```python
from build123d import *

# Parameters (mm, degrees)
M3_SFHCS_IN_HAV_A1_D           = 3.4
M3_SFHCS_IN_HAV_A1_CSINK_D     = 6.72
M3_SFHCS_IN_HAV_A1_CSINK_ANGLE = 90
DAIRESEL_KAPLAMA1_COUNT        = 10


with BuildPart() as part:
    # Çizim1 → Döndür2 (revolve)
    with BuildSketch(Plane.XY, mode=Mode.PRIVATE) as d_nd_r2_sk:
        with BuildLine():
            Line((26.6, -13.648391358), (26.6, -3.648391358))
            Line((26.6, -3.648391358), (25.1, -3.648391358))
            Line((25.1, -3.648391358), (25.1, 4.751608642))
            ThreePointArc((25.1, 4.751608642), (30.108474042, 16.843134601), (42.2, 21.851608642))
            Line((42.2, 21.851608642), (55.5, 21.851608642))
            ThreePointArc((55.5, 21.851608642), (60.449747468, 23.901861174), (62.5, 28.851608642))
            Line((62.5, 28.851608642), (62.5, 53.351608642))
            Line((62.5, 53.351608642), (64, 53.351608642))
            Line((64, 53.351608642), (64, 61.351608642))
            Line((64, 61.351608642), (66, 61.351608642))
            Line((66, 61.351608642), (66, 51.351608642))
            Line((66, 51.351608642), (64.5, 51.351608642))
            Line((64.5, 51.351608642), (64.5, 18.851608642))
            Line((64.5, 18.851608642), (39.98, 18.851608642))
            ThreePointArc((39.98, 18.851608642), (31.57957144, 15.372037203), (28.1, 6.971608642))
            Line((28.1, 6.971608642), (28.1, -13.648391358))
            Line((28.1, -13.648391358), (26.6, -13.648391358))
        make_face()
    revolve(d_nd_r2_sk.sketch.rotate(Axis((0, 0, 0), (0, 1, 0)), 90), axis=Axis((0, 0, 0), (0, 1, 0)))

    # M3 SFHCS İçin Havşa1 (through all)
    with Locations(Plane(origin=(8.5, 18.851608642, 50.5), x_dir=(0, 0, -1), z_dir=(0, -1, 0))):
        with Locations((0, 0)):
            m3_sfhcs_in_hav_a1 = CounterSinkHole(M3_SFHCS_IN_HAV_A1_D / 2, M3_SFHCS_IN_HAV_A1_CSINK_D / 2, counter_sink_angle=M3_SFHCS_IN_HAV_A1_CSINK_ANGLE)

    # Dairesel Kaplama1: M3 SFHCS İçin Havşa1 ×10 about axis
    dairesel_kaplama1_axis = Axis((0, 0, 0), (0, 1, 0))
    for i in range(1, DAIRESEL_KAPLAMA1_COUNT):
        add(m3_sfhcs_in_hav_a1.rotate(dairesel_kaplama1_axis, i * 360 / DAIRESEL_KAPLAMA1_COUNT), mode=Mode.SUBTRACT)


solid = part.part
```
Read the model definition and answer for the solid it produces. Units are mm, in the model's axes. A direction names the side the tool comes from. Give positions to 0.01 mm unless a question says otherwise; leave off trailing zeros. Order: outer loops, then holes, each group sorted by start corner. A loop starts at its lowest first (then second) coordinate and runs counter-clockwise, first axis right, second up.
(1) Straight lines are drawn through the part: L1, parallel to X at y = 40.5, z = 0; L2, parallel to X at y = 0.5, z = 0; L3, parallel to Y at x = 30, z = 40. For each, find the intervals that lie inside material, in ascending order.
(2) Given pin 1 (12 mm diameter, centred on x = 46, z = -50, fed in from +Y); pin 2 (3 mm diameter, centred on x = -45.4, z = 23.69, fed in from -Y); pin 3 (4 mm diameter, centred on x = 45.4, z = -23.69, fed in from +Y); pin 4 (1.5 mm diameter, centred on x = -39, z = 16, fed in from -Y), each flat-ended and moving along its own axis, determine where each tip first touches the part or whether it passes through.
(3) Find section D-D (y = 34.5). Give the vertices of the cut face in (x, z), plus the area to 3 significant figures.
(4) For faces 4 (the cylindrical face through (-2.75, 41.27, 62.44)), 5 (the cylindrical face through (9.613, 0.61, -23.186)), 6 (the flat face through (14.4, 51.352, -63.2)), determine the directions among +Z, -Z, +X, -X, +Y, -Y from which every point of the face is accessible in a straight line to the end or side of a thin tool.
(5) Find section C-C (y = -7). Give the vertices of the cut face in (x, z), plus the area to 3 significant figures.
(6) For a pull along X with two mould halves and no side action, classify faces 1 (the cylindrical face through (-24.488, 21.191, 45.6)), 2 (the cylindrical face through (-19.825, 56.282, -62.952)), 3 (the flat face through (28, 18.852, 30)) as released by +X, released by -X, zero draft, split by the parting line, or undercut.
Result sheet:
1. L1: x = -64.5 to -62.5, 62.5 to 64.5
1. L2: x = -28.1 to -25.1, 25.1 to 28.1
1. L3: y = 18.85 to 21.85
2. pin 1: stops at y = 61.35
2. pin 2: passes through
2. pin 3: stops at y = 21.85
2. pin 4: stops at y = 18.85
3. outline: circle Ø129 at (0, 0); hole circle Ø125 at (0, 0)
3. area: 798 mm2
4. face 4: +Y
4. face 5: +Y, -Y
4. face 6: -Y
5. outline: circle Ø56.2 at (0, 0); hole circle Ø53.2 at (0, 0)
5. area: 258 mm2
6. face 1: undercut
6. face 2: split by the parting line
6. face 3: zero draft
